Source: CAD feature listing. Evaluate the final solid. Frame: model axes, mm. A direction names the side the tool comes from. Round coordinates to 2 decimals unless told otherwise and drop trailing zeros. Write each loop counter-clockwise with the first axis right and the second up, starting at its lowest first coordinate (ties: lowest second). Pieces come first, ordered by that corner, then holes. Notation, with made-up numbers: M 79.25,65 L 114.25,65 A26 cw 114.25,97 Z; hole C 35.5,23 d4. An arc over 180 degrees is marked long. Use a Markdown table: item, result.
```python
from build123d import *

# Parameters (mm, degrees)
F0_W     = 127.219696
F0_H     = 77.92443
F1_DEPTH = 7.62
F2_R     = 6.034431
F3_DEPTH = 38.1


with BuildPart() as f1:
    # F0 (on Top) → F1 (new body)
    with BuildSketch(Plane.XY):
        with Locations((8.437073, -9.764254)):
            Rectangle(F0_W, F0_H)
    extrude(amount=F1_DEPTH)

    # F2 (on Top) → F3 (join)
    with BuildSketch(Plane.XY):
        with Locations((-47.020096, -40.952984)):
            Circle(F2_R)
        with Locations((-47.155522, 21.089828)):
            Circle(F2_R)
        with Locations((64.309441, -40.952984)):
            Circle(F2_R)
        with Locations((64.309441, 21.089828)):
            Circle(F2_R)
    extrude(amount=F3_DEPTH)


solid = f1.part
```
Q1. Section D-D on x = 6.5. Return loops of the section in (y, z).
Results are:
| item | result |
|---|---|
| outline | M -48.73,0 L 29.2,0 L 29.2,7.62 L -48.73,7.62 Z |
Q2. Section C-C on z = 15. Return loops of the section in (x, y).
Results are:
| item | result |
|---|---|
| outline | C -47.16,21.09 d12.07; C -47.02,-40.95 d12.07; C 64.31,-40.95 d12.07; C 64.31,21.09 d12.07 |
Q3. Section A-A on y = 19.5. Return loops of the section in (x, z).
Results are:
| item | result |
|---|---|
| outline | M -55.17,0 L 72.05,0 L 72.05,7.62 L 70.13,7.62 L 70.13,38.1 L 58.49,38.1 L 58.49,7.62 L -41.33,7.62 L -41.33,38.1 L -52.98,38.1 L -52.98,7.62 L -55.17,7.62 Z |
Q4. Mould query, pull axis X, two halves, no side actions, for faces 3 (the flat face through (-47, -41, 38.1)), 4 (the cylindrical face through (59.862, 25.168, 22.647)), 5 (the flat face through (-55.173, -10, 4)), 6 (the flat face through (8, -9, 7.62)). Classes: +X half, -X half, draft (parallel to the pull), parting line (faces both ways), or undercut.
Results are:
| item | result |
|---|---|
| face 3 | draft |
| face 4 | undercut |
| face 5 | -X half |
| face 6 | undercut |
Q5. Section B-B on x = -47. Return loops of the section in (y, z).
Results are:
| item | result |
|---|---|
| outline | M -48.73,0 L 29.2,0 L 29.2,7.62 L 27.12,7.62 L 27.12,38.1 L 15.06,38.1 L 15.06,7.62 L -34.92,7.62 L -34.92,38.1 L -46.99,38.1 L -46.99,7.62 L -48.73,7.62 Z |
Q6. Line query: L1, parallel to Y at x = -47.5, z = 32; L2, parallel to Z at x = -9, y = -45; L3, parallel to Y at x = 65, z = 27. Output: solid intervals per line, ascending.
Results are:
| item | result |
|---|---|
| L1 | -46.97 to -34.94, 15.07 to 27.11 |
| L2 | 0 to 7.62 |
| L3 | -46.95 to -34.96, 15.1 to 27.08 |
Q7. Reachability of faces 1 (the cylindrical face through (59.862, -36.875, 22.647)), 2 (the flat face through (8, 29.198, 4)) from +Z, -Z, +X, -X, +Y, -Y: full face, straight path, thin tool, end or side. Return the list, or none.
Results are:
| item | result |
|---|---|
| face 1 | +Z |
| face 2 | +Z, -Z, +X, -X, +Y |
Q8. First-contact query: pin 1 Ø1 at (y, z) = (15, 18.5) entering from +X; pin 2 Ø8 at (y, z) = (20, 15.5) entering from -X; pin 3 Ø6 at (y, z) = (-7, 11) entering from +X; pin 4 Ø6 at (y, z) = (18, 26.5) entering from +X. Flat tips, straight axial feed; report the tip coordinate or a pass-through.
Results are:
| item | result |
|---|---|
| pin 1 | x = 66.58 |
| pin 2 | x = -53.19 |
| pin 3 | through |
| pin 4 | x = 70.34 |
